Check sheet for the modelled part. Datum: model origin and axes. Units: mm. A direction names the side the tool comes from. Round coordinates to 2 decimals unless told otherwise and drop trailing zeros. Write each loop counter-clockwise with the first axis right and the second up, starting at its lowest first coordinate (ties: lowest second). Pieces come first, ordered by that corner, then holes. Notation, with made-up numbers: (54, 7.25) - (105, 7.25) arc R28 ccw to (105, 38.25) - close; hole circle Ø9 at (44, -29). An arc over 180 degrees is marked (long way). Answer as a JSON object with one key per item and string values. Group by question number.
Item 1: Sectioned sample at C-C on z = 9. Record the boundary of the cut face in (x, y).
Item 2: Thickness scan on line 1 (Z direction, x = 12.5, y = 2.5); line 2 (X direction, y = -1.5, z = 53); line 3 (Z direction, x = -16, y = -3). Record the ranges inside material, lowest first.
Item 3: Sectioned sample at D-D on x = -15.5. Record the boundary of the cut face in (y, z), plus the area to 3 significant figures.
Item 4: Sectioned sample at A-A on y = 2.25. Record the boundary of the cut face in (x, z), plus the area to 3 significant figures.
Item 5: Sectioned sample at B-B on x = 7. Record the boundary of the cut face in (y, z).
Item 6: Set-up check for faces 5 (the flat face through (0, 3.55, 1)), 6 (the flat face through (2.915, 2, 54)), 7 (the flat face through (33.02, -1, -1)): record each of +Z, -Z, +X, -X, +Y, -Y from which the full face is reachable in a straight line by a thin tool's end or side.
Item 7: Gauge pin test, flat ends, axial feed: P1, Ø0.5, axis at y = -1, z = -64, coming from the +X side; P2, Ø0.5, axis at y = -0.5, z = -64, coming from the -X side; P3, Ø2, axis at x = 20.5, z = -48.5, coming from the -Y side. Record the tip position at first contact, or that the pin passes through.
Item 8: Release check for a two-part mould opening along Y. For faces 1 (the cylindrical face through (34.11, -0.05, -63.62)), 2 (the flat face through (0, -1.748, -64)), 3 (the flat face through (0, 1.01, 1)), 4 (the flat face through (0, 0, -64)) record: pulls with the +Y half, pulls with the -Y half, needs draft (parallel to the pull), parting line crosses it, or undercut.
```python
from build123d import *

# Parameters (mm, degrees)
F0_W     = 71.120002
F0_H     = 130.28951
F1_DEPTH = 3.55
F2_T     = -2.54
F3_R     = 5.08
F4_W     = 28.56459
F4_H     = 12.824923
F5_DEPTH = 12.5
F6_W     = 10.341828
F6_H     = 1.748307
F7_DEPTH = 12.5


with BuildPart() as f1:
    # F0 (on Front) → F1 (new body, symmetric)
    with BuildSketch(Plane.XZ):
        Rectangle(F0_W, F0_H)
    extrude(amount=F1_DEPTH, both=True)

    # F2
    f2_openings = [f1.faces().sort_by_distance(p)[0] for p in [
        (0, -3.55, 0),
    ]]
    offset(amount=F2_T, openings=f2_openings)

    # F3
    f3_edges = [f1.edges().sort_by_distance(p)[0] for p in [
        (35.560001, 0, 65.144755),
        (-35.560001, 0, 65.144755),
        (35.560001, 0, -65.144755),
        (-35.560001, 0, -65.144755),
    ]]
    fillet(f3_edges, radius=F3_R)

    # F4 (on face) → F5 (cut, symmetric)
    with BuildSketch(Plane.XZ.offset(-1.01)):
        with Locations((17.19705, 54.360166)):
            Rectangle(F4_W, F4_H)
    extrude(amount=F5_DEPTH, both=True, mode=Mode.SUBTRACT)

    # F6 (on face) → F7 (cut, symmetric)
    with BuildSketch(Plane(origin=(0, 0, -65.144755), x_dir=(1, 0, 0), z_dir=(0, 0, -1))):
        with Locations((0, 0.874153)):
            Rectangle(F6_W, F6_H)
    extrude(amount=F7_DEPTH, both=True, mode=Mode.SUBTRACT)


solid = f1.part
```
Completed:
{
 "1": {"outline": "(-35.56, -3.55) - (-33.02, -3.55) - (-33.02, 1.01) - (33.02, 1.01) - (33.02, -3.55) - (35.56, -3.55) - (35.56, 3.55) - (-35.56, 3.55) - close"},
 "2": {"line 1": "-65.14 to 47.95, 60.77 to 65.14", "line 2": "-35.56 to -33.02, 33.02 to 35.56", "line 3": "-65.14 to -62.6, 62.6 to 65.14"},
 "3": {"outline": "(-3.55, -65.14) - (3.55, -65.14) - (3.55, 65.14) - (-3.55, 65.14) - (-3.55, 62.6) - (1.01, 62.6) - (1.01, -62.6) - (-3.55, -62.6) - close", "area": "354 mm²"},
 "4": {"outline": "(-35.56, -60.06) arc R5.08 ccw to (-30.48, -65.14) - (30.48, -65.14) arc R5.08 ccw to (35.56, -60.06) - (35.56, 60.06) arc R5.08 ccw to (30.48, 65.14) - (-30.48, 65.14) arc R5.08 ccw to (-35.56, 60.06) - close; hole (2.91, 47.95) - (31.48, 47.95) - (31.48, 60.77) - (2.91, 60.77) - close", "area": "8,880 mm²"},
 "5": {"outline": "(-3.55, -65.14) - (3.55, -65.14) - (3.55, 47.95) - (1.01, 47.95) - (1.01, -62.6) - (-3.55, -62.6) - close; (-3.55, 62.6) - (1.01, 62.6) - (1.01, 60.77) - (3.55, 60.77) - (3.55, 65.14) - (-3.55, 65.14) - close"},
 "6": {"face 5": "+Z, -Z, +X, -X, +Y", "face 6": "+Y, -Y", "face 7": "-Y"},
 "7": {"P1": "x = 33.98", "P2": "x = -33.98", "P3": "y = 1.01"},
 "8": {"face 1": "needs draft", "face 2": "undercut", "face 3": "pulls with the -Y half", "face 4": "undercut"}
}
